from build123d import *

# Parameters (mm, degrees)
SKETCH1_W           = 42
SKETCH1_H           = 25
BOSS_EXTRUDE1_DEPTH = 60
CUT_EXTRUDE1_DEPTH  = 56
SKETCH3_R           = 4
CUT_EXTRUDE2_DEPTH  = 15


with BuildPart() as part:
    # Sketch1 → Boss-Extrude1 (new body)
    with BuildSketch(Plane(origin=(0, 0, 0), x_dir=(1, 0, 0), z_dir=(0, 1, 0))):
        with Locations((21, 12.5)):
            Rectangle(SKETCH1_W, SKETCH1_H)
    extrude(amount=BOSS_EXTRUDE1_DEPTH)

    # Sketch2 → Cut-Extrude1 (cut)
    with BuildSketch(Plane.XY):
        with BuildLine():
            Line((42, 40), (21, 40))
            ThreePointArc((21, 40), (11, 30), (21, 20))
            Line((21, 20), (42, 20))
            Line((42, 20), (42, 40))
        make_face()
    extrude(amount=-CUT_EXTRUDE1_DEPTH, mode=Mode.SUBTRACT)

    # Sketch3 → Cut-Extrude2 (cut)
    with BuildSketch(Plane(origin=(42, 0, 0), x_dir=(0, 0, -1), z_dir=(1, 0, 0))):
        with Locations((12.5, 10)):
            Circle(SKETCH3_R)
        with Locations(Location((12.5, 50, 0), (0, 0, 180))):
            Circle(SKETCH3_R)
    extrude(amount=-CUT_EXTRUDE2_DEPTH, mode=Mode.SUBTRACT)


solid = part.part
Design review of the part built by this model. Coordinates are the model's own, in mm. A direction names the side the tool comes from. Give positions to 0.01 mm unless a question says otherwise; leave off trailing zeros. Write each loop counter-clockwise with the first axis right and the second up, starting at its lowest first coordinate (ties: lowest second). Pieces come first, ordered by that corner, then holes. Notation, with made-up numbers: M -27,29.25 L 8,29.25 A24 ccw 8,45.25 Z; hole C -22.5,36 d6. An arc over 180 degrees is marked long. Answer as a JSON object with one key per item and string values. Group by question number.
1) We need section A-A (x = 28.5). Give the boundary of the cut face in (y, z).
2) We need section B-B (y = 50). Give the boundary of the cut face in (x, z), and give its area (3 significant figures).
3) Clearance check with a flat-ended pin moving along its axis: pin 1 Ø2 at (y, z) = (30, -18.5) entering from -X. State where the tip first meets the part, or that it passes through.
4) Mouldability with a two-part tool opening along Z and no side actions: class faces 4 (the face through (11, 30, -12)), 5 (the face through (11, 36, -25)), 6 (the face through (27, 10, -12)) as released by +Z, released by -Z, zero draft, split by the parting line, or undercut.
5) We need section D-D (z = -12.5). Give the boundary of the cut face in (x, y).
6) We need section C-C (x = 13.5). Give the boundary of the cut face in (y, z), and give its area (3 significant figures).
7) For line 1 along Y through (x, z) = (32.5, -12.5); line 2 along Z through (x, y) = (36.25, 50); line 3 along Y through (x, z) = (40.5, -5.5), list the stretches that pass through material, from the lowest coordinate up.
8) Tool access review of faces 1 (the face through (21, 60, -13)), 2 (the face through (34.6, 52.4, -15.7)), 3 (the face through (32, 40, -12)): name each direction out of +Z, -Z, +X, -X, +Y, -Y from which nothing blocks a thin tool from reaching the whole face with its end or side.
Answer key:
{
 "1": {"outline": "M 0,-25 L 20,-25 L 20,0 L 0,0 Z; M 40,-25 L 60,-25 L 60,0 L 40,0 Z; hole C 10,-12.5 d8; hole C 50,-12.5 d8"},
 "2": {"outline": "M 0,-25 L 42,-25 L 42,-16.5 L 27,-16.5 L 27,-8.5 L 42,-8.5 L 42,0 L 0,0 Z", "area": "930 mm²"},
 "3": {"pin 1": "stops at x = 0"},
 "4": {"face 4": "zero draft", "face 5": "released by -Z", "face 6": "undercut"},
 "5": {"outline": "M 0,0 L 42,0 L 42,6 L 27,6 L 27,14 L 42,14 L 42,20 L 21,20 A10 cw 21,40 L 42,40 L 42,46 L 27,46 L 27,54 L 42,54 L 42,60 L 0,60 Z"},
 "6": {"outline": "M 0,-25 L 23.39,-25 L 23.39,0 L 0,0 Z; M 36.61,-25 L 60,-25 L 60,0 L 36.61,0 Z", "area": "1,170 mm²"},
 "7": {"line 1": "y = 0 to 6, 14 to 20, 40 to 46, 54 to 60", "line 2": "z = -25 to -16.5, -8.5 to 0", "line 3": "y = 0 to 20, 40 to 60"},
 "8": {"face 1": "+Z, -Z, +X, -X, +Y", "face 2": "+X", "face 3": "+Z, -Z, +X"}
}
